Autodesk Inventor part; units mm, degrees
ref_plane "YZ Plane" through (0, 0, 0) normal (1, 0, 0) x (0, 1, 0)
ref_plane "XZ Plane" through (0, 0, 0) normal (0, 1, 0) x (-1, 0, 0)
ref_plane "XY Plane" through (0, 0, 0) normal (0, 0, 1) x (1, 0, 0)
sketch "Sketch1" plane through (0, 0, 0) normal (0, 0, 1) x (1, 0, 0)
  line L0 (0, 0) -> (0, 18.35)
  line L1 (0, 0) -> (-12, 0)
  line L2 (-12, 0) -> (-12, 3)
  line L3 (-12, 3) -> (-10, 3)
  line L4 (-10, 3) -> (-10, 18.35)
  line L5 (-10, 18.35) -> (0, 18.35)
  dimension "d0" = 20
  dimension "d1" = 24
  dimension "d2" = 3
  dimension "d3" = 18.35
revolve "Revolution1" add sketch "Sketch1" angle 360 about axis through (0, 0, 0) along (0, 1, 0)
sketch "Sketch2" plane through (0, 0, 0) normal (0, -1, 0) x (1, 0, 0)
  point P0 (0, 0)
  point P1 (0, 0)
  point P2 (6, 0)
  point P3 (-6, 0)
  dimension "d6" = 6
  dimension "d7" = 6
hole "Hole1" at (0, 0, 0) at (6, 0, 0) at (-6, 0, 0) direction (0, 1, 0) diameter 3 end through all counterbore diameter 5 counterbore depth 15
sketch "Sketch3" plane through (0, 0, 0) normal (0, -1, 0) x (1, 0, 0)
  line L0 (-15, 1) -> (15, 1)
  line L1 (15, 1) -> (15, -1)
  line L2 (15, -1) -> (-15, -1)
  line L3 (-15, -1) -> (-15, 1)
  line L4 (-15, 1) -> (15, -1) construction
  line L5 (15, 1) -> (-15, -1) construction
  point P0 (0, 0)
  dimension "d15" = 30
  dimension "d16" = 2
extrude "Extrusion1" cut sketch "Sketch3" against normal blind 2
properties part number "019" material "PAEK Plastic"
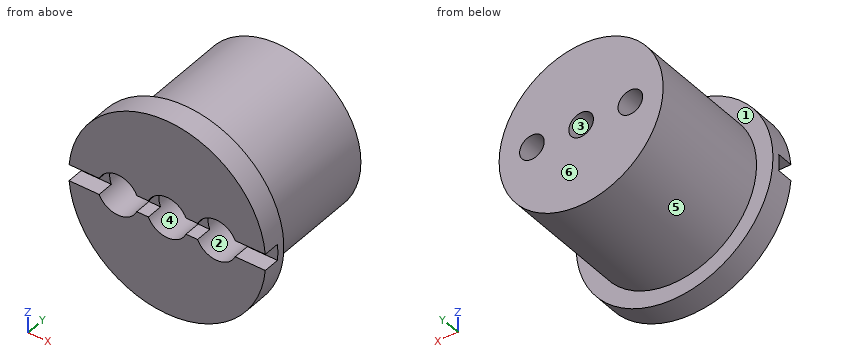
Source: CAD feature listing. Evaluate the final solid. Frame: model axes, mm. Face numbers are marked on the shaded views. A direction names the side the tool comes from. Give positions to 0.01 mm unless a question says otherwise; leave off trailing zeros. Write each loop counter-clockwise with the first axis right and the second up, starting at its lowest first coordinate (ties: lowest second). Pieces come first, ordered by that corner, then holes. Notation, with made-up numbers: (11, 9.25) -> (40, 9.25) arc R7 cw to (40, 18.25) -> close; hole circle Ø9 at (66, 21). An arc over 180 degrees is marked (long way). Return JSON: item names as keys, results as strings. Group by question number.
1. Material intervals for line 1 (Z direction, x = 0, y = 10.5); line 2 (Y direction, x = 3, z = 10.75); line 3 (X direction, y = 9, z = 0.75), sorted ascending. Write a range as from..to.
2. Mould query, pull axis X, two halves, no side actions, for the marked faces 4, 5 and 6. Classes: +X half, -X half, draft (parallel to the pull), parting line (faces both ways), or undercut.
3. Section D-D, the plane y = 11.5. Output: boundary loops of the cut face in (x, z), then the cut area to 3 significant figures.
4. Section B-B, the plane x = 0. Output: boundary loops of the cut face in (y, z), then the cut area to 3 significant figures.
5. Pin query (flat end, axial travel): pin 1 Ø1.6 at (x, z) = (-2.5, 0) entering from -Y; pin 2 Ø0.6 at (x, y) = (10.5, 0.5) entering from +Z; pin 3 Ø3 at (x, y) = (8.5, 13) entering from -Z. Return the tip coordinate at first contact, or that it passes through.
6. Access query for the marked faces 1, 2 and 3. Directions: +Z, -Z, +X, -X, +Y, -Y. A direction counts if a zero-diameter tool reaches every point of the face in a straight line with its end or side. Return the directions, or none.
7. Section C-C, the plane y = 1.5. Output: boundary loops of the cut face in (x, z).
8. Section A-A, the plane z = 0. Count the separate pieces of the cut face and the enclosed holes in it, then the cut area to 3 significant figures.
Determined:
{
 "1": {"line 1": "z = -10..-2.5, 2.5..10", "line 2": "y = 0..3", "line 3": "x = -9.97..-8.38, -3.62..-2.38, 2.38..3.62, 8.38..9.97"},
 "2": {"face 4": "undercut", "face 5": "parting line", "face 6": "draft"},
 "3": {"outline": "circle Ø20 at (0, 0); hole circle Ø5 at (-6, 0); hole circle Ø5 at (0, 0); hole circle Ø5 at (6, 0)", "area": "255 mm2"},
 "4": {"outline": "(0, -12) -> (3, -12) -> (3, -10) -> (18.35, -10) -> (18.35, -1.5) -> (15, -1.5) -> (15, -2.5) -> (0, -2.5) -> close; (0, 2.5) -> (15, 2.5) -> (15, 1.5) -> (18.35, 1.5) -> (18.35, 10) -> (3, 10) -> (3, 12) -> (0, 12) -> close", "area": "294 mm2"},
 "5": {"pin 1": "stops at y = 2", "pin 2": "stops at z = 6.32", "pin 3": "stops at z = -7.14"},
 "6": {"face 1": "+Y", "face 2": "-Y", "face 3": "+Y, -Y"},
 "7": {"outline": "(-11.96, -1) arc R12 ccw to (11.96, -1) -> (8.29, -1) arc R2.5 cw to (3.71, -1) -> (2.29, -1) arc R2.5 cw to (-2.29, -1) -> (-3.71, -1) arc R2.5 cw to (-8.29, -1) -> close; (-11.96, 1) -> (-8.29, 1) arc R2.5 cw to (-3.71, 1) -> (-2.29, 1) arc R2.5 cw to (2.29, 1) -> (3.71, 1) arc R2.5 cw to (8.29, 1) -> (11.96, 1) arc R12 ccw to start"},
 "8": {"separate pieces": "4", "enclosed holes": "0", "area": "106 mm2"}
}
